```python
from build123d import *

# Parameters (mm, degrees)
SKETCH1_W           = 254
SKETCH1_H           = 203.2
BOSS_EXTRUDE1_DEPTH = 6.35
SKETCH2_R           = 4.7498
CUT_EXTRUDE2_DEPTH  = 6.35


with BuildPart() as part:
    # Sketch1 → Boss-Extrude1 (new body)
    with BuildSketch(Plane.XY):
        Rectangle(SKETCH1_W, SKETCH1_H)
    extrude(amount=BOSS_EXTRUDE1_DEPTH)

    # Sketch2 → Cut-Extrude2 (cut)
    with BuildSketch(Plane.XY.offset(6.35)):
        with Locations((114.3, -90.297)):
            Circle(SKETCH2_R)
        with Locations(Location((-114.3, -90.297, 0), (0, 0, 180))):
            Circle(SKETCH2_R)
        with Locations(Location((114.3, 90.297, 0), (0, 0, 180))):
            Circle(SKETCH2_R)
        with Locations((-114.3, 90.297)):
            Circle(SKETCH2_R)
    extrude(amount=-CUT_EXTRUDE2_DEPTH, mode=Mode.SUBTRACT)


solid = part.part
```
The listing builds one solid part. Answer for the finished solid, in the listing's coordinates (mm). Give positions to 0.01 mm unless a question says otherwise; leave off trailing zeros. Write each loop counter-clockwise with the first axis right and the second up, starting at its lowest first coordinate (ties: lowest second). Pieces come first, ordered by that corner, then holes. Notation, with made-up numbers: M 88.25,69.25 L 146.25,69.25 A19 cw 146.25,101.25 Z; hole C -31,80 d8. An arc over 180 degrees is marked long. Write each question's results on one line, items separated by ' | '.
Q1. For a pull along X with two mould halves and no side action, classify faces 1 (the cylindrical face through (109.77, 88.87, 3.22)), 2 (the flat face through (127, -1, 3)), 3 (the flat face through (-127, -1, 3)), 4 (the flat face through (-2, -101.6, 3)) as released by +X, released by -X, zero draft, split by the parting line, or undercut.
Output values:
face 1: undercut | face 2: released by +X | face 3: released by -X | face 4: zero draft
Q2. Consider L1, parallel to Y at x = -114.3, z = 3; L2, parallel to X at y = -86, z = 1.75; L3, parallel to X at y = 89, z = 4.25. Determine where each line is inside the solid, lowest interval first. Write a range as from..to.
Output values:
L1: -101.6..-95.05, -85.55..85.55, 95.05..101.6 | L2: -127..-116.32, -112.28..112.28, 116.32..127 | L3: -127..-118.87, -109.73..109.73, 118.87..127
Q3. Section A-A, the plane x = 114.3 is taken. Write down the section's boundary in (y, z), then the cut area to 3 significant figures.
Output values:
outline: M -101.6,0 L -95.05,0 L -95.05,6.35 L -101.6,6.35 Z; M -85.55,0 L 85.55,0 L 85.55,6.35 L -85.55,6.35 Z; M 95.05,0 L 101.6,0 L 101.6,6.35 L 95.05,6.35 Z | area: 1,170 mm2
